```python
from build123d import *

# Parameters (mm, degrees)
SKETCH1_W                    = 101.6
SKETCH1_H                    = 101.6
EXTRUDE1_DEPTH               = 3.175
SKETCH2_W                    = 101.6
SKETCH2_H                    = 3.175
EXTRUDE2_DEPTH               = 101.6
FILLET1_R                    = 12.7
SKETCH3_R                    = 9.525
EXTRUDE3_DEPTH               = 61.9125
F_97_0_0059_DIAMETER_HOLE1_D = 6.35
SKETCH7_R                    = 38.1
SKETCH7_W                    = 76.2
SKETCH7_H                    = 44.45
EXTRUDE4_DEPTH               = 47.625
SKETCH10_R                   = 36.5125
EXTRUDE12_DEPTH              = 101.6


with BuildPart() as part:
    # Sketch1 → Extrude1 (new body)
    with BuildSketch(Plane(origin=(0, 0, 0), x_dir=(1, 0, 0), z_dir=(0, 1, 0))):
        Rectangle(SKETCH1_W, SKETCH1_H)
    extrude(amount=EXTRUDE1_DEPTH)

    # Sketch2 → Extrude2 (add)
    with BuildSketch(Plane(origin=(0, 3.175, 0), x_dir=(1, 0, 0), z_dir=(0, 1, 0))):
        with Locations((0, -49.2125)):
            Rectangle(SKETCH2_W, SKETCH2_H)
    extrude(amount=EXTRUDE2_DEPTH)

    # Fillet1
    fillet1_edges = [part.edges().sort_by_distance(p)[0] for p in [
        (0, 3.175, 47.625),
    ]]
    fillet(fillet1_edges, radius=FILLET1_R)

    # Sketch3 → Extrude3 (add)
    with BuildSketch(Plane.XY.offset(50.8)):
        with Locations(Location((0, 52.3875, 0), (0, 0, 180))):
            Circle(SKETCH3_R)
    extrude(amount=EXTRUDE3_DEPTH)

    # #97 (0.0059) Diameter Hole1 (through all)
    with Locations(Plane(origin=(0, 3.175, 0), x_dir=(-1, 0, 0), z_dir=(0, 1, 0))):
        with Locations((-25.4, 25.4), (25.4, 25.4), (25.4, -25.4), (-25.4, -25.4)):
            Hole(F_97_0_0059_DIAMETER_HOLE1_D / 2)

    # Sketch7 → Extrude4 (add)
    with BuildSketch(Plane(origin=(0, 0, 47.625), x_dir=(-1, 0, 0), z_dir=(0, 0, -1))):
        with Locations((0, 52.3875)):
            Circle(SKETCH7_R)
        with Locations((0, 74.6125)):
            Rectangle(SKETCH7_W, SKETCH7_H)
    extrude(amount=EXTRUDE4_DEPTH)

    # Sketch10 → Extrude12 (add)
    with BuildSketch(Plane(origin=(38.1, 0, 0), x_dir=(0, 0, -1), z_dir=(1, 0, 0))):
        with Locations(Location((-9.525, 79.375, 0), (0, 0, 227.657394548))):
            Circle(SKETCH10_R)
    extrude(amount=EXTRUDE12_DEPTH)


solid = part.part
```
Verification items for the finished model (mm, model axes). A direction names the side the tool comes from. Give positions to 0.01 mm unless a question says otherwise; leave off trailing zeros. Order: outer loops, then holes, each group sorted by start corner. A loop starts at its lowest first (then second) coordinate and runs counter-clockwise, first axis right, second up. Notation, with made-up numbers: M -17,-21 L 32,-21 A22 ccw 32,-1 Z; hole C -14,11 d5. An arc over 180 degrees is marked long. Return JSON: item names as keys, results as strings. Group by question number.
1) Section check C-C on z = 9. Record the cut outline in (x, y) (1 decimal).
2) Scan lines: line 1 (Z direction, x = -25, y = 1); line 2 (Z direction, x = 25.4, y = 1.2) (3 decimals); line 3 (Y direction, x = 14.5, z = -25) (3 decimals). Record each from-to range of solid material in increasing order.
3) Mould release check, pull along Y, two halves, no side actions. Record for faces 1 (the face through (-1, 99, 47.625)), 2 (the face through (1.24, 42.944, 81.323)), 3 (the face through (-1, 0, -1)), 4 (the face through (1, 56, 0)): pulls with the +Y half, pulls with the -Y half, needs draft (parallel to the pull), parting line crosses it, or undercut.
4) Section check D-D on y = 83. Record the cut outline in (x, z) (3 decimals), and give its area (3 significant figures).
5) Access from +Z, -Z, +X, -X, +Y, -Y to the whole of each face (thin tool, end or side, straight path). Record for faces 5 (the face through (-1, 3.175, -9)), 6 (the face through (-38.1, 74, 24)), 7 (the face through (50.8, 29, 49)), 8 (the face through (28.43, 1.57, 26.35)), 9 (the face through (38.1, 68, 45)).
6) Section check A-A on x = 47. Record the cut outline in (y, z) (1 decimal).
7) Go/stop test with flat-tipped pins: pin 1 Ø10 at (x, z) = (-25.4, -25.4) entering from +Y (3 decimals); pin 2 Ø5 at (y, z) = (43, 57.5) entering from +X; pin 3 Ø5 at (x, y) = (44, 22) entering from -Z (3 decimals); pin 4 Ø4 at (x, z) = (25.4, -25.4) entering from -Y. Record where each tip stops, or that it passes through.
8) Section check B-B on x = -25.4. Record the cut outline in (y, z) (1 decimal), and give its area (3 significant figures).
Answer block:
{
 "1": {"outline": "M -50.8,0 L 50.8,0 L 50.8,3.2 L -50.8,3.2 Z; M -38.1,52.4 A38.1 ccw 38.1,52.4 L 38.1,42.9 L 139.7,42.9 L 139.7,115.9 L 38.1,115.9 L 38.1,96.8 L -38.1,96.8 Z"},
 "2": {"line 1": "z = -50.8 to -28.55, -22.25 to 22.25, 28.55 to 50.8", "line 2": "z = -50.8 to -28.575, -22.225 to 22.225, 28.575 to 50.8", "line 3": "y = 0 to 3.175"},
 "3": {"face 1": "undercut", "face 2": "parting line crosses it", "face 3": "pulls with the -Y half", "face 4": "needs draft"},
 "4": {"outline": "M -50.8,47.625 L -38.1,47.625 L -38.1,0 L 38.1,0 L 38.1,-26.807 L 139.7,-26.807 L 139.7,45.857 L 38.1,45.857 L 38.1,47.625 L 50.8,47.625 L 50.8,50.8 L -50.8,50.8 Z", "area": "11,300 mm^2"},
 "5": {"face 5": "-Z, +X, -X", "face 6": "-Z, -X, +Y", "face 7": "+Z, +X, -Y", "face 8": "-Y", "face 9": "+X"},
 "6": {"outline": "M 0,-50.8 L 3.2,-50.8 L 3.2,34.9 A12.7 cw 15.9,47.6 L 104.8,47.6 L 104.8,50.8 L 0,50.8 Z; C 79.4,9.5 d73"},
 "7": {"pin 1": "stops at y = 3.175", "pin 2": "stops at x = 6.58", "pin 3": "stops at z = 47.625", "pin 4": "passes through"},
 "8": {"outline": "M 0,-50.8 L 3.2,-50.8 L 3.2,-28.6 L 0,-28.6 Z; M 0,-22.2 L 3.2,-22.2 L 3.2,22.2 L 0,22.2 Z; M 0,28.6 L 3.2,28.6 L 3.2,34.9 A12.7 cw 15.9,47.6 L 24,47.6 L 24,0 L 96.8,0 L 96.8,47.6 L 104.8,47.6 L 104.8,50.8 L 0,50.8 Z", "area": "4,110 mm^2"}
}
